from build123d import *

# Parameters (mm, degrees)
EXTRUDE_1_DEPTH          = 8
SKETCH_2_R               = 20
CUT_EXTRUDE_1_DEPTH      = 9
HOLE_WIZARD_M3_1_D       = 3.6
PATTERN_CIRCULAR_1_COUNT = 8
CHAMFER_1_SIZE           = 1
HOLE_WIZARD_M4_1_D       = 4.5
CUT_EXTRUDE_2_DEPTH      = 3.3
SKETCH_8_R               = 21
CUT_EXTRUDE_3_DEPTH      = 7


with BuildPart() as part:
    # ｽｹｯﾁ1 → ﾎﾞｽ - 押し出し1 (new body)
    with BuildSketch(Plane.XY):
        with BuildLine():
            Line((31, -31), (-31, -31))
            Line((-31, -31), (-31, 0))
            ThreePointArc((-31, 0), (0, 31), (31, 0))
            Line((31, 0), (31, -31))
        make_face()
    extrude(amount=EXTRUDE_1_DEPTH)

    # ｽｹｯﾁ2 → ｶｯﾄ - 押し出し1 (cut, through all)
    with BuildSketch(Plane.XY.offset(8)):
        Circle(SKETCH_2_R)
    extrude(amount=-CUT_EXTRUDE_1_DEPTH, mode=Mode.SUBTRACT)

    # M3 すきま穴1 (through all)
    with Locations(Plane.XY.offset(8)):
        with Locations((0, 27.5)):
            hole_wizard_m3_1 = Hole(HOLE_WIZARD_M3_1_D / 2)

    # 円形ﾊﾟﾀｰﾝ1: M3 すきま穴1 ×8 about axis
    pattern_circular_1_axis = Axis((0, 0, 0), (0, 0, 1))
    for i in range(1, PATTERN_CIRCULAR_1_COUNT):
        add(hole_wizard_m3_1.rotate(pattern_circular_1_axis, i * 360 / PATTERN_CIRCULAR_1_COUNT), mode=Mode.SUBTRACT)

    # 面取り1
    chamfer_1_edges = [part.edges().sort_by_distance(p)[0] for p in [
        (31, -15.5, 0),
        (0, -31, 0),
        (-31, -15.5, 0),
        (0, 31, 0),
        (31, -31, 4),
        (-31, -31, 4),
    ]]
    chamfer(chamfer_1_edges, length=CHAMFER_1_SIZE)

    # M4 すきま穴1 (through all)
    with Locations(Plane.XY.offset(8)):
        with Locations((-27.5, -21), (27.5, -21)):
            Hole(HOLE_WIZARD_M4_1_D / 2)

    # ｽｹｯﾁ7 → ｶｯﾄ - 押し出し2 (cut)
    with BuildSketch(Plane.XY):
        Polygon((-27.5, -25.041451884), (-24, -23.020725942), (-24, -18.979274058), (-27.5, -16.958548116), (-31, -18.979274058), (-31, -23.020725942), align=None)
        Polygon((31, -18.979274058), (27.5, -16.958548116), (24, -18.979274058), (24, -23.020725942), (27.5, -25.041451884), (31, -23.020725942), align=None)
    extrude(amount=CUT_EXTRUDE_2_DEPTH, mode=Mode.SUBTRACT)

    # ｽｹｯﾁ8 → ｶｯﾄ - 押し出し3 (cut)
    with BuildSketch(Plane(origin=(0, 0, 8), x_dir=(-1, 0, 0), z_dir=(0, 0, -1))):
        Circle(SKETCH_8_R)
    extrude(amount=CUT_EXTRUDE_3_DEPTH, mode=Mode.SUBTRACT)


solid = part.part
For this review, take the finished solid that the model builds, in its own axes (mm). A direction names the side the tool comes from. Coordinates: 2 decimals unless noted, no trailing zeros. Loops run counter-clockwise (first coordinate to the right, second up) from the corner with the lowest first, then second, coordinate; pieces in that order, holes last. Notation, with made-up numbers: (76.5, 72.5) -> (99.5, 72.5) arc R22 ccw to (99.5, 94.5) -> close; hole circle Ø3 at (89, 52). An arc over 180 degrees is marked (long way). Write each question's results on one line, items separated by ' | '.
Q1. Add section D-D, the plane y = -10. State the section outline as (x, z) points, then the cut area to 3 significant figures.
Taken from the geometry:
outline: (-31, 1) -> (-30, 0) -> (-17.32, 0) -> (-17.32, 1) -> (-18.47, 1) -> (-18.47, 8) -> (-31, 8) -> close; (17.32, 0) -> (30, 0) -> (31, 1) -> (31, 8) -> (18.47, 8) -> (18.47, 1) -> (17.32, 1) -> close | area: 202 mm²
Q2. Machinability: for faces 1 (the flat face through (25.7, -24, 1.6)), 2 (the flat face through (-24, -21, 2)), 3 (the cylindrical face through (-20.03, 6.31, 4.55)), which of the approach directions +Z, -Z, +X, -X, +Y, -Y give a long, thin tool a straight path to every point of the face, cutting with its end or side? Answer none if there is none.
Taken from the geometry:
face 1: -Z | face 2: -Z, -X | face 3: +Z
Q3. Add section C-C, the plane z = 6.5. Count the separate pieces of the cut face and the enclosed holes in it, then the cut area to 3 significant figures.
Taken from the geometry:
separate pieces: 1 | enclosed holes: 11 | area: 1,930 mm²
Q4. Add section A-A, the plane x = 0. State the section outline as (y, z) points.
Taken from the geometry:
outline: (-31, 1) -> (-30, 0) -> (-29.3, 0) -> (-29.3, 8) -> (-31, 8) -> close; (-25.7, 0) -> (-20, 0) -> (-20, 1) -> (-21, 1) -> (-21, 8) -> (-25.7, 8) -> close; (20, 0) -> (25.7, 0) -> (25.7, 8) -> (21, 8) -> (21, 1) -> (20, 1) -> close; (29.3, 0) -> (30, 0) -> (31, 1) -> (31, 8) -> (29.3, 8) -> close
Q5. For pin 1 Ø3 at (x, y) = (0, -27.5) entering from +Z; pin 2 Ø2.5 at (y, z) = (-21.5, 1) entering from -X; pin 3 Ø5 at (x, y) = (27.5, -21) entering from +Z; pin 4 Ø4 at (y, z) = (12.5, 6) entering from -X, all flat-tipped, find the tip position at first contact; note any pin that passes through.
Taken from the geometry:
pin 1: through | pin 2: x = -24 | pin 3: z = 8 | pin 4: x = -29.17
Q6. Add section B-B, the plane y = -27.5. State the section outline as (x, z) points, then the cut area to 3 significant figures.
Taken from the geometry:
outline: (-31, 1) -> (-30, 0) -> (-1.8, 0) -> (-1.8, 8) -> (-31, 8) -> close; (1.8, 0) -> (30, 0) -> (31, 1) -> (31, 8) -> (1.8, 8) -> close | area: 466 mm²
Q7. Mouldability with a two-part tool opening along Y and no side actions: class faces 4 (the cylindrical face through (19.368, -21.244, 3.944)), 5 (the flat face through (31, -15, 4)) as +Y half, -Y half, draft (parallel to the pull), parting line (faces both ways), or undercut.
Taken from the geometry:
face 4: undercut | face 5: draft
Q8. To check wall thickness, follow line 1 along Y through (x, z) = (0, 6); line 2 along Y through (x, z) = (0, 0.6); line 3 along X through (y, z) = (18, 4.5). State the ranges of each line that lie inside material, in increasing order. Write a range as [from, to].
Taken from the geometry:
line 1: [-31, -29.3], [-25.7, -21], [21, 25.7], [29.3, 31] | line 2: [-30.6, -29.3], [-25.7, -20], [20, 25.7], [29.3, 30.6] | line 3: [-25.24, -20.52], [-18.37, -10.82], [10.82, 18.37], [20.52, 25.24]
